Can you work these out from the model? Positions are in its coordinate system, mm. A direction names the side the tool comes from. Coordinates: 2 decimals unless noted, no trailing zeros. Loops run counter-clockwise (first coordinate to the right, second up) from the corner with the lowest first, then second, coordinate; pieces in that order, holes last. Notation, with made-up numbers: (-34, 73) -> (19, 73) arc R14 cw to (19, 91) -> close; hole circle Ø7 at (-5, 30). An arc over 180 degrees is marked (long way). Put each result on its own line as item: value. Start each with the question number.
Item 1: Will these pins go through, and if not, where does the flat tip stop? P1, Ø1.2, axis at y = 5.5, z = 93.5, coming from the -X side; P2, Ø3, axis at x = 0, z = 83, coming from the +Y side; P3, Ø1.5, axis at y = 2, z = -20, coming from the -X side.
Item 2: If we section it at A-A on z = -102.5: Please give me the cut outline in (x, y).
Item 3: We'd pull the mould along X, two halves only. Please class faces 5 (the cylindrical face through (35.827, 1.521, 100.584)), 6 (the flat face through (22, 5, -87)), 7 (the flat face through (33, 5, -64)): pulls with the +X half, pulls with the -X half, needs draft (parallel to the pull), parting line crosses it, or undercut.
Item 4: Please list where these lines run through material, in increasing order: L1, parallel to Z at x = 24.5, y = 6.25; L2, parallel to X at y = 0.95, z = 49.5; L3, parallel to X at y = 0.95, z = -49.5. Write a range as from..to.
Item 5: If we section it at B-B on y = 1.5: State how many separate pieces and enclosed holes the cut face has, plus the area to 3 significant figures.
Item 6: For faces 1 (the flat face through (0, 5, 65)), 2 (the flat face through (8, 5, -94)), 3 (the flat face through (-22, 5, 77.5)), 4 (the flat face through (8, 5, -1)), which set-ups out of +Z, -Z, +X, -X, +Y, -Y let a thin tool reach every point of the face, with its end or its side?
Item 7: If we section it at D-D on z = 49.5: Please give me the cut outline in (x, y).
```python
from build123d import *

# Parameters (mm, degrees)
BOSS_EXTRUDE1_DEPTH          = 3
SKETCH2_R                    = 2.6
CUT_EXTRUDE1_DEPTH           = 115.890534423
CIRPATTERN1_COUNT            = 2
SKETCH4_W                    = 3
SKETCH4_H                    = 100
BOSS_EXTRUDE2_DEPTH          = 4
BOSS_EXTRUDE3_START          = -4
SKETCH5_W                    = 70
SKETCH5_H                    = 3
BOSS_EXTRUDE3_DEPTH          = 4
CHAMFER2_SIZE                = 4
CIRPATTERN2_COUNT            = 2
CHAMFER2_OF_CIRPATTERN2_SIZE = 4


with BuildPart() as part:
    # Sketch1 → Boss-Extrude1 (new body)
    with BuildSketch(Plane(origin=(0, 0, 0), x_dir=(1, 0, 0), z_dir=(0, 1, 0))):
        Polygon((39.57, -44.5), (39.57, -107.5), (-40.43, -107.5), (-40.43, -44.5), (-15, -44.5), (-15, 44.5), (-39.57, 44.5), (-39.57, 107.5), (40.43, 107.5), (40.43, 44.5), (15, 44.5), (15, -44.5), align=None)
    extrude(amount=BOSS_EXTRUDE1_DEPTH)

    # Sketch2 → Cut-Extrude1 (cut, through all)
    with BuildSketch(Plane(origin=(0, 3, 0), x_dir=(1, 0, 0), z_dir=(0, 1, 0))):
        with Locations(Location((20.07, -49.5, 0), (0, 0, 270))):
            Circle(SKETCH2_R)
        with Locations(Location((34.07, -49.5, 0), (0, 0, 270))):
            Circle(SKETCH2_R)
        with Locations(Location((34.07, -102.5, 0), (0, 0, 270))):
            Circle(SKETCH2_R)
        with Locations(Location((20.07, -102.5, 0), (0, 0, 270))):
            Circle(SKETCH2_R)
        with Locations(Location((-14.68, -49.5, 0), (0, 0, 270))):
            Circle(SKETCH2_R)
        with Locations(Location((-27.18, -49.5, 0), (0, 0, 270))):
            Circle(SKETCH2_R)
        with Locations(Location((-14.68, -102.5, 0), (0, 0, 270))):
            Circle(SKETCH2_R)
        with Locations(Location((-27.18, -102.5, 0), (0, 0, 270))):
            Circle(SKETCH2_R)
    cut_extrude1 = extrude(amount=-CUT_EXTRUDE1_DEPTH, mode=Mode.SUBTRACT)

    # CirPattern1: Cut-Extrude1 ×2 about axis
    cirpattern1_axis = Axis((0, 0, 0), (0, 1, 0))
    for i in range(1, CIRPATTERN1_COUNT):
        add(cut_extrude1.rotate(cirpattern1_axis, i * 360 / CIRPATTERN1_COUNT), mode=Mode.SUBTRACT)

    # Sketch4 → Boss-Extrude2 (add)
    with BuildSketch(Plane(origin=(0, 3, 0), x_dir=(1, 0, 0), z_dir=(0, 1, 0))):
        with Locations((6.5, -50)):
            Rectangle(SKETCH4_W, SKETCH4_H)
        with Locations((-6.5, -50)):
            Rectangle(SKETCH4_W, SKETCH4_H)
    boss_extrude2 = extrude(amount=BOSS_EXTRUDE2_DEPTH)

    # Sketch5 → Boss-Extrude3 (add)
    with BuildSketch(Plane(origin=(0, 7, 0), x_dir=(1, 0, 0), z_dir=(0, 1, 0)).offset(BOSS_EXTRUDE3_START)):
        with Locations((0, -88.5)):
            Rectangle(SKETCH5_W, SKETCH5_H)
        with Locations((0, -63.5)):
            Rectangle(SKETCH5_W, SKETCH5_H)
        with Locations((0, -76)):
            Rectangle(SKETCH5_W, SKETCH5_H)
    boss_extrude3 = extrude(amount=BOSS_EXTRUDE3_DEPTH)

    # Chamfer2
    chamfer2_edges = [part.edges().sort_by_distance(p)[0] for p in [
        (35, 7, 63.5),
        (35, 7, 76),
        (35, 7, 88.5),
        (6.5, 7, 100),
        (-6.5, 7, 100),
        (-35, 7, 88.5),
        (-35, 7, 76),
        (-35, 7, 63.5),
    ]]
    chamfer(chamfer2_edges, length=CHAMFER2_SIZE - 0.0001)  # a hair under: the kernel refuses the full size

    # CirPattern2: Boss-Extrude2, Boss-Extrude3 ×2 about axis
    cirpattern2_axis = Axis((0, 0, 0), (0, 1, 0))
    add([boss_extrude2.rotate(cirpattern2_axis, i * 360 / CIRPATTERN2_COUNT) for i in range(1, CIRPATTERN2_COUNT)])
    add([boss_extrude3.rotate(cirpattern2_axis, i * 360 / CIRPATTERN2_COUNT) for i in range(1, CIRPATTERN2_COUNT)])

    # Chamfer2 of CirPattern2
    chamfer2_of_cirpattern2_edges = [part.edges().sort_by_distance(p)[0] for p in [
        (-35, 7, -63.5),
        (-35, 7, -76),
        (-35, 7, -88.5),
        (-6.5, 7, -100),
        (6.5, 7, -100),
        (35, 7, -88.5),
        (35, 7, -76),
        (35, 7, -63.5),
    ]]
    chamfer(chamfer2_of_cirpattern2_edges, length=CHAMFER2_OF_CIRPATTERN2_SIZE - 0.0001)  # a hair under: the kernel refuses the full size


solid = part.part
```
Solutions:
1. P1: x = -8
1. P2: y = 3
1. P3: x = -15
2. outline: (-39.57, 0) -> (-36.67, 0) -> (-36.67, 3) -> (-39.57, 3) -> close; (-31.47, 0) -> (-22.67, 0) -> (-22.67, 3) -> (-31.47, 3) -> close; (-17.47, 0) -> (12.08, 0) -> (12.08, 3) -> (-17.47, 3) -> close; (17.28, 0) -> (24.58, 0) -> (24.58, 3) -> (17.28, 3) -> close; (29.78, 0) -> (40.43, 0) -> (40.43, 3) -> (29.78, 3) -> close
3. face 5: undercut
3. face 6: needs draft
3. face 7: pulls with the +X half
4. L1: -90..-87, -77.5..-74.5, -65..-62, 62..65, 74.5..77.5, 87..90
4. L2: -40.43..-29.78, -24.58..-17.28, -12.08..17.47, 22.67..31.47, 36.67..39.57
4. L3: -39.57..-36.67, -31.47..-22.67, -17.47..12.08, 17.28..24.58, 29.78..40.43
5. separate pieces: 1
5. enclosed holes: 16
5. area: 12,400 mm^2
6. face 1: +Y
6. face 2: -Z, +X, +Y
6. face 3: -X, +Y
6. face 4: +X, +Y
7. outline: (-40.43, 0) -> (-29.78, 0) -> (-29.78, 3) -> (-40.43, 3) -> close; (-24.58, 0) -> (-17.28, 0) -> (-17.28, 3) -> (-24.58, 3) -> close; (-12.08, 0) -> (17.47, 0) -> (17.47, 3) -> (8, 3) -> (8, 7) -> (5, 7) -> (5, 3) -> (-5, 3) -> (-5, 7) -> (-8, 7) -> (-8, 3) -> (-12.08, 3) -> close; (22.67, 0) -> (31.47, 0) -> (31.47, 3) -> (22.67, 3) -> close; (36.67, 0) -> (39.57, 0) -> (39.57, 3) -> (36.67, 3) -> close
